Source: CAD feature listing. Evaluate the final solid. Frame: model axes, mm. Coordinates: 2 decimals unless noted, no trailing zeros. Write each loop counter-clockwise with the first axis right and the second up, starting at its lowest first coordinate (ties: lowest second). Pieces come first, ordered by that corner, then holes. Notation, with made-up numbers: (36, -11) - (46, -11) arc R21 ccw to (46, 27) - close; hole circle Ø11 at (21, -32.75). An arc over 180 degrees is marked (long way). One line per item, written item: value.
Autodesk Inventor part; units mm, degrees
ref_plane "YZ Plane" through (0, 0, 0) normal (1, 0, 0) x (0, 1, 0)
ref_plane "XZ Plane" through (0, 0, 0) normal (0, 1, 0) x (-1, 0, 0)
ref_plane "XY Plane" through (0, 0, 0) normal (0, 0, 1) x (1, 0, 0)
sketch "Sketch1" plane through (0, 0, 0) normal (0, 0, 1) x (1, 0, 0)
  line L0 (-20.5, -20.5) -> (20.5, -20.5)
  line L1 (20.5, -20.5) -> (20.5, 20.5)
  line L2 (20.5, 20.5) -> (-20.5, 20.5)
  line L3 (-20.5, 20.5) -> (-20.5, -20.5)
  line L4 (-20.5, -20.5) -> (20.5, 20.5) construction
  line L5 (20.5, -20.5) -> (-20.5, 20.5) construction
  point P0 (0, 0)
  dimension "d0" = 41
  dimension "d1" = 41
extrude "Extrusion1" add sketch "Sketch1" along normal blind 4
sketch "Sketch2" plane through (0, 0, 4) normal (0, 0, 1) x (1, 0, 0)
  circle A0 centre (0, 0) radius 5.5
  dimension "d4" = 11
extrude "Extrusion2" cut sketch "Sketch2" against normal blind 4
sketch "Sketch3" plane through (0, 0, 4) normal (0, 0, 1) x (1, 0, 0)
  circle A0 centre (0, 0) radius 5.5
  circle A1 centre (0, 0) radius 6.45
  circle A2 centre (-18.375, 0) radius 2.125
  circle A3 centre (18.375, 0) radius 2.125
  line L0 (-18.721, 2.0966) -> (-4.7075, 4.4093)
  line L1 (-18.7594, -2.0899) -> (-4.3799, -4.7348)
  line L2 (18.7217, 2.0965) -> (4.702, 4.4152)
  line L3 (18.7594, -2.0899) -> (4.3799, -4.7348)
  line L4 (0, 0) -> (18.375, 0)
  line L5 (0, 0) -> (-18.375, 0)
  circle A4 centre (-14.175, -4.4) radius 1.15
  circle A5 centre (14.175, 4.4) radius 1.15
  dimension "d7" = 12.9
  dimension "d8" = 4.25
  dimension "d9" = 4.25
  dimension "d10" = 9.15
  dimension "d11" = 9.15
  dimension "d12" = 41
  dimension "d13" = 18.375
  dimension "d14" = 2.3
  dimension "d15" = 4.4
  dimension "d16" = 4.2
  dimension "d17" = 2.3
  dimension "d18" = 4.4
  dimension "d19" = 4.2
extrude "Extrusion3" cut sketch "Sketch3" against normal blind 4 contours A4 | A5
mirror "Mirror1" about plane through (0, 0, 0) normal (0, 1, 0) of "Extrusion3"
pattern_circular "Circular Pattern1" count 4 over 360 about axis through (0, 0, 4) along (0, 0, -1) of "Extrusion3", "Mirror1"
properties part number "servo_attachment"
1) Material intervals for line 1 (X direction, y = 4.4, z = 2.5) (3 decimals); line 2 (Y direction, x = -14.5, z = 0.6); line 3 (X direction, y = 4.5, z = 1.5), sorted ascending.
Values found:
line 1: -20.5 to -15.325, -13.025 to -3.3, 3.3 to 13.025, 15.325 to 20.5
line 2: -20.5 to -5.5, -3.3 to 3.3, 5.5 to 20.5
line 3: -20.5 to -15.32, -13.03 to -3.16, 3.16 to 13.03, 15.32 to 20.5
2) Section query C-C on x = -4.4. Output: boundary loops of the cut face in (y, z) (3 decimals), then the cut area to 3 significant figures.
Values found:
outline: (-20.5, 0) - (-15.325, 0) - (-15.325, 4) - (-20.5, 4) - close; (-13.025, 0) - (-3.3, 0) - (-3.3, 4) - (-13.025, 4) - close; (3.3, 0) - (13.025, 0) - (13.025, 4) - (3.3, 4) - close; (15.325, 0) - (20.5, 0) - (20.5, 4) - (15.325, 4) - close
area: 119 mm2
3) Draft query along X for faces 1 (the flat face through (0, 20.5, 2)), 2 (the cylindrical face through (13.026, 4.451, 2.028)), 3 (the flat face through (-20.5, 0, 2)). Return one class per face: released by +X, released by -X, zero draft, split by the parting line, or undercut.
Values found:
face 1: zero draft
face 2: undercut
face 3: released by -X
4) Section query A-A on x = 0. Output: boundary loops of the cut face in (y, z), then the cut area to 3 significant figures.
Values found:
outline: (-20.5, 0) - (-5.5, 0) - (-5.5, 4) - (-20.5, 4) - close; (5.5, 0) - (20.5, 0) - (20.5, 4) - (5.5, 4) - close
area: 120 mm2
